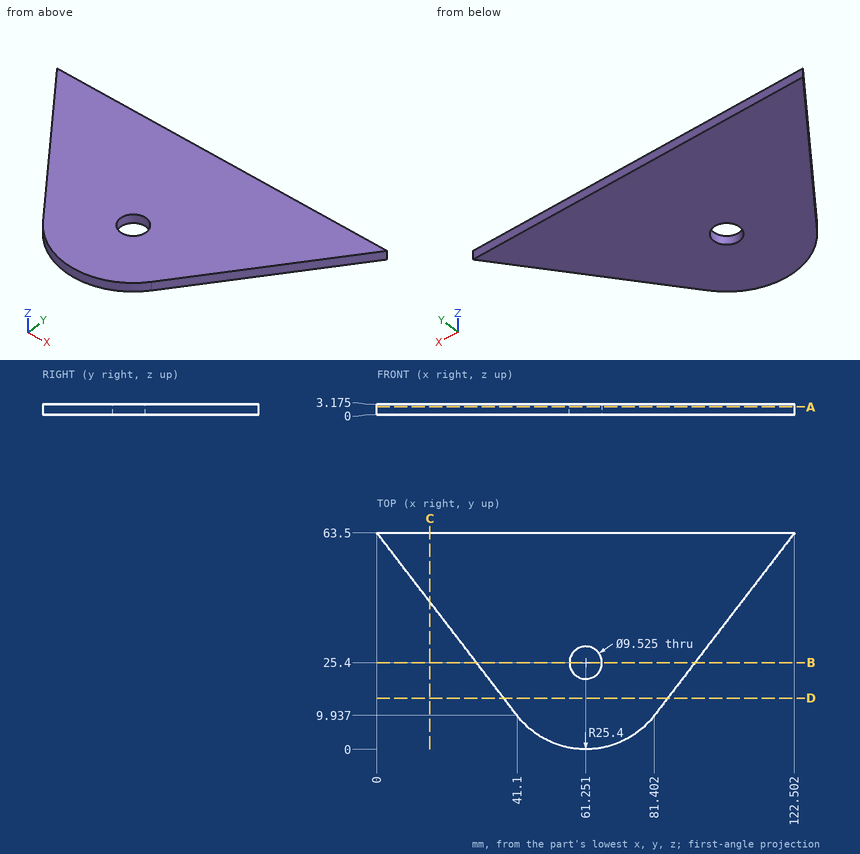
Can you work these out from the drawing? Everything is in mm from the part's minimum corner. Round coordinates to 2 decimals unless told otherwise and drop trailing zeros. Write each loop counter-clockwise with the first axis right and the second up, starting at its lowest first coordinate (ties: lowest second). Pieces come first, ordered by that corner, then holes. Notation, with made-up numbers: M 79,48.5 L 116,48.5 A12 cw 116,68.5 Z; hole C 54,-21.75 d1. An arc over 180 degrees is marked long. Use a Markdown table: item, result.
Item 1: I want a section at C-C (x = 15.5). List the corners of the cut face in (y, z) for me (1 decimal).
Found:
| item | result |
|---|---|
| outline | M 43.3,0 L 63.5,0 L 63.5,3.2 L 43.3,3.2 Z |
Item 2: For pin 1 Ø1.5 at (x, z) = (35, 1.5) entering from -Y, with a flat end and sliding along its axis, tell me the tip position at first contact or that it passes through.
Found:
| item | result |
|---|---|
| pin 1 | stops at y = 16.91 |
Item 3: I want a section at A-A (z = 2.3). List the corners of the cut face in (x, y) for me (1 decimal).
Found:
| item | result |
|---|---|
| outline | M 0,63.5 L 41.1,9.9 A25.4 ccw 81.4,9.9 L 122.5,63.5 Z; hole C 61.3,25.4 d9.5 |
Item 4: If I drill on line 1 along X through (y, z) = (28.5, 0.15) (1 decimal); line 2 along X through (y, z) = (29, 1.25) (1 decimal); line 3 along Y through (x, z) = (60, 2) (1 decimal), over which ranges is the centre line in solid material (lowest first)? Write a range as [from, to].
Found:
| item | result |
|---|---|
| line 1 | x = [26.9, 57.6], [64.9, 95.6] |
| line 2 | x = [26.5, 58.1], [64.4, 96] |
| line 3 | y = [0, 20.8], [30, 63.5] |
Item 5: I want a section at D-D (y = 15). List the corners of the cut face in (x, z) for me (1 decimal), and give its area (3 significant figures).
Found:
| item | result |
|---|---|
| outline | M 37.2,0 L 85.3,0 L 85.3,3.2 L 37.2,3.2 Z |
| area | 153 mm2 |
Item 6: I want a section at B-B (y = 25.4). List the corners of the cut face in (x, z) for me (1 decimal).
Found:
| item | result |
|---|---|
| outline | M 29.2,0 L 56.5,0 L 56.5,3.2 L 29.2,3.2 Z; M 66,0 L 93.3,0 L 93.3,3.2 L 66,3.2 Z |
